Part model, mm, in its own coordinate system. Face numbers are marked on the shaded views. A direction names the side the tool comes from. Round coordinates to 2 decimals unless told otherwise and drop trailing zeros. Loops run counter-clockwise (first coordinate to the right, second up) from the corner with the lowest first, then second, coordinate; pieces in that order, holes last. Notation, with made-up numbers: M 15,-2.5 L 45,-2.5 A24 cw 45,31.5 Z; hole C -32,-34.75 d3. An arc over 180 degrees is marked long. Put each result on its own line as item: value. Start each with the question number.
```python
from build123d import *

# Parameters (mm, degrees)
SKETCH1_W           = 200
SKETCH1_H           = 200
BOSS_EXTRUDE1_DEPTH = 10
SKETCH2_W           = 175
SKETCH2_H           = 175
BOSS_EXTRUDE2_DEPTH = 75
CUT_EXTRUDE2_DEPTH  = 188.5
SKETCH6_W           = 50.093360238
SKETCH6_H           = 155
CUT_EXTRUDE3_DEPTH  = 100
SKETCH7_R           = 10
BOSS_EXTRUDE4_DEPTH = 100


with BuildPart() as part:
    # Sketch1 → Boss-Extrude1 (new body)
    with BuildSketch(Plane.XY):
        Rectangle(SKETCH1_W, SKETCH1_H)
    extrude(amount=BOSS_EXTRUDE1_DEPTH)

    # Sketch2 → Boss-Extrude2 (add)
    with BuildSketch(Plane(origin=(0, 0, 0), x_dir=(-1, 0, 0), z_dir=(0, 0, -1))):
        Rectangle(SKETCH2_W, SKETCH2_H)
    extrude(amount=BOSS_EXTRUDE2_DEPTH)

    # Sketch5 → Cut-Extrude2 (cut, through all)
    with BuildSketch(Plane(origin=(0, 87.5, 0), x_dir=(1, 0, 0), z_dir=(0, 1, 0))):
        with BuildLine():
            Line((-87.5, 0), (-53.713488753, 60))
            ThreePointArc((-53.713488753, 60), (-50.046464226, 63.72662143), (-45, 65.093360238))
            Line((-45, 65.093360238), (45, 65.093360238))
            ThreePointArc((45, 65.093360238), (50.046464226, 63.72662143), (53.713488753, 60))
            Line((53.713488753, 60), (87.5, 0))
            Line((87.5, 0), (87.5, 75))
            Line((87.5, 75), (-87.5, 75))
            Line((-87.5, 75), (-87.5, 0))
        make_face()
    extrude(amount=-CUT_EXTRUDE2_DEPTH, mode=Mode.SUBTRACT)

    # Sketch6 → Cut-Extrude3 (cut, symmetric)
    with BuildSketch(Plane(origin=(0, 0, 0), x_dir=(0, 0, -1), z_dir=(1, 0, 0))):
        with Locations((40.046680119, 0)):
            Rectangle(SKETCH6_W, SKETCH6_H)
    extrude(amount=CUT_EXTRUDE3_DEPTH, both=True, mode=Mode.SUBTRACT)

    # Sketch7 → Boss-Extrude4 (add, symmetric)
    with BuildSketch(Plane(origin=(0, 0, 0), x_dir=(1, 0, 0), z_dir=(0, 1, 0))):
        with Locations((0, 50)):
            Circle(SKETCH7_R)
    extrude(amount=BOSS_EXTRUDE4_DEPTH, both=True)


solid = part.part
```
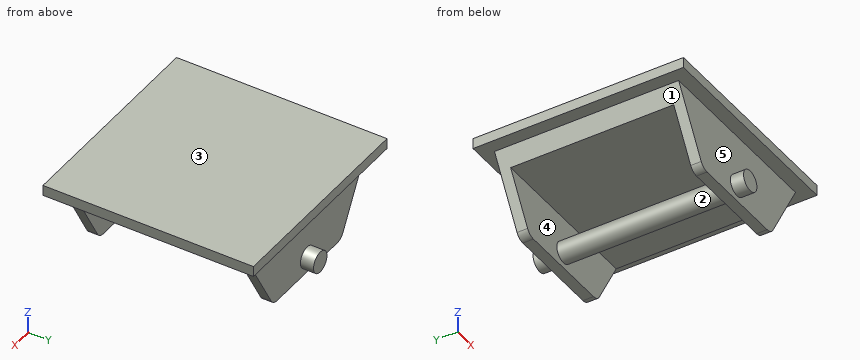
1. Cut at C-C, the plane z = -56. Give the cut face in (x, y), and give its area (3 significant figures).
2. Cut at B-B, the plane x = -19. Give the cut face in (y, z).
3. Wall check: L1, parallel to Z at x = 0, y = 43.5; L2, parallel to Z at x = -68, y = 23; L3, parallel to Y at x = -50, z = -57.5. Give the ranges that are in metal, low to high.
4. Drop flat-ended pins along their axis: pin 1 (12 mm diameter, centred on y = -14, z = -49.5, fed in from +X); pin 2 (6 mm diameter, centred on x = 14.5, z = -1, fed in from -Y); pin 3 (1.5 mm diameter, centred on x = -28.5, z = -47, fed in from -Y); pin 4 (12 mm diameter, centred on y = -10, z = -50, fed in from -X). Give the stop position or say it passes through.
5. Cut at A-A, the plane y = 14. Give the cut face in (x, z), and give its area (3 significant figures).
6. Mould opens along Y. For the marked faces 3, 4 and 5 say: released by +Y, released by -Y, zero draft, split by the parting line, or undercut.
7. Cut at D-D, the plane x = -61.5. Give the cut face in (y, z), and give its area (3 significant figures).
8. Which spindle directions (+Z, -Z, +X, -X, +Y, -Y) get a long thin tool onto all of the face, cutting with end or side? Do the marked faces 1 and 2. Say none if no direction does.
Results list:
1. outline: M -55.97,-87.5 L -8,-87.5 L -8,-100 L 8,-100 L 8,-87.5 L 55.97,-87.5 L 55.97,-77.5 L 8,-77.5 L 8,77.5 L 55.97,77.5 L 55.97,87.5 L 8,87.5 L 8,100 L -8,100 L -8,87.5 L -55.97,87.5 L -55.97,77.5 L -8,77.5 L -8,-77.5 L -55.97,-77.5 Z
1. area: 5,120 mm^2
2. outline: M -100,0 L -87.5,0 L -87.5,-65.09 L -77.5,-65.09 L -77.5,-15 L 77.5,-15 L 77.5,-65.09 L 87.5,-65.09 L 87.5,0 L 100,0 L 100,10 L -100,10 Z
3. L1: z = -60 to -40, -15 to 10
3. L2: z = -15 to 10
3. L3: y = -87.5 to -77.5, 77.5 to 87.5
4. pin 1: stops at x = 10
4. pin 2: stops at y = -100
4. pin 3: stops at y = -87.5
4. pin 4: stops at x = -10
5. outline: M -100,0 L -87.5,0 L -79.05,-15 L 79.05,-15 L 87.5,0 L 100,0 L 100,10 L -100,10 Z; C 0,-50 d20
5. area: 4,810 mm^2
6. face 3: zero draft
6. face 4: undercut
6. face 5: released by -Y
7. outline: M -100,0 L -87.5,0 L -87.5,-46.17 L -77.5,-46.17 L -77.5,-15 L 77.5,-15 L 77.5,-46.17 L 87.5,-46.17 L 87.5,0 L 100,0 L 100,10 L -100,10 Z
7. area: 5,250 mm^2
8. face 1: -Z, -X, +Y, -Y
8. face 2: none
